Read the model definition and answer for the solid it produces. Units are mm, in the model's axes. Coordinates: 2 decimals unless noted, no trailing zeros. Order: outer loops, then holes, each group sorted by start corner. A loop starts at its lowest first (then second) coordinate and runs counter-clockwise, first axis right, second up. Notation, with made-up numbers: M 11,81.5 L 44,81.5 A22 cw 44,90.5 Z; hole C 51,-4.75 d9. An arc over 180 degrees is marked long. Use a Markdown table: item, result. Add a question column.
1) Find the intervals of material crossed by probe 1 along Y at (x, z) = (0, 22.75); probe 2 along X at (y, z) = (-40, 9.5); probe 3 along Y at (x, z) = (36.5, 10.25), in increasing order. Write a range as [from, to].
2) Find section B-B on x = -29.5. Write down the section's boundary in (y, z), plus the area to 3 significant figures.
3) Find section A-A on z = 3.75. Write down the section's boundary in (x, y), plus the area to 3 significant figures.
4) The mould has two halves that part along Y. Classify faces 1 (the face through (-43.3, 0.1, 14.8)), 2 (the face through (1.2, -20, 15)), 3 (the face through (-3, 0, 0)): released by +Y, released by -Y, zero draft, split by the parting line, or undercut.
5) Each of these flat-tipped pins is pushed along its axis until it touches: pin 1 Ø5 at (x, z) = (6.5, 17) entering from -Y; pin 2 Ø1 at (y, z) = (16.5, 24.5) entering from -X; pin 3 Ø12 at (y, z) = (10, 12.5) entering from +X. Where does it stop, or does it pass through?
from build123d import *

# Parameters (mm, degrees)
BOSS_EXTRUDE1_DEPTH = 30
SKETCH1_3_R         = 0.9
CUT_EXTRUDE1_DEPTH  = 30


with BuildPart() as part:
    # Sketch1 → Boss-Extrude1 (new body)
    with BuildSketch(Plane.XY):
        with BuildLine():
            Line((-1.2, -1.2), (-1.2, 0))
            Line((-1.2, 0), (-1.2, 1.2))
            Line((-1.2, 1.2), (-3.07408523, 1.2))
            ThreePointArc((-3.07408523, 1.2), (-3.3, 0), (-3.07408523, -1.2))
            Line((-3.07408523, -1.2), (-1.2, -1.2))
        make_face()
        with BuildLine():
            ThreePointArc((0, -1.2), (-0.848528137, -0.848528137), (-1.2, 0))
            Line((-1.2, 0), (-1.2, -1.2))
            Line((-1.2, -1.2), (0, -1.2))
        make_face()
        with BuildLine():
            ThreePointArc((0, 1.2), (-0.848528137, 0.848528137), (-1.2, 0))
            ThreePointArc((-1.2, 0), (-0.848528137, -0.848528137), (0, -1.2))
            ThreePointArc((0, -1.2), (0.848528137, -0.848528137), (1.2, 0))
            ThreePointArc((1.2, 0), (0.848528137, 0.848528137), (0, 1.2))
        make_face()
        with BuildLine():
            Line((-1.2, 1.2), (-1.2, 0))
            ThreePointArc((-1.2, 0), (-0.848528137, 0.848528137), (0, 1.2))
            Line((0, 1.2), (-1.2, 1.2))
        make_face()
        with BuildLine():
            Line((-3.07408523, 1.2), (-1.2, 1.2))
            Line((-1.2, 1.2), (-1.2, 3.07408523))
            ThreePointArc((-1.2, 3.07408523), (-2.333452378, 2.333452378), (-3.07408523, 1.2))
        make_face()
        with BuildLine():
            Line((-1.2, 3.07408523), (-1.2, 1.2))
            Line((-1.2, 1.2), (0, 1.2))
            Line((0, 1.2), (1.2, 1.2))
            Line((1.2, 1.2), (1.2, 3.07408523))
            ThreePointArc((1.2, 3.07408523), (0, 3.3), (-1.2, 3.07408523))
        make_face()
        with BuildLine():
            Line((0, -1.2), (-1.2, -1.2))
            Line((-1.2, -1.2), (-1.2, -3.07408523))
            ThreePointArc((-1.2, -3.07408523), (0, -3.3), (1.2, -3.07408523))
            Line((1.2, -3.07408523), (1.2, -1.2))
            Line((1.2, -1.2), (0, -1.2))
        make_face()
        with BuildLine():
            Line((-1.2, -3.07408523), (-1.2, -1.2))
            Line((-1.2, -1.2), (-3.07408523, -1.2))
            ThreePointArc((-3.07408523, -1.2), (-2.333452378, -2.333452378), (-1.2, -3.07408523))
        make_face()
        with BuildLine():
            ThreePointArc((1.2, 0), (0.848528137, -0.848528137), (0, -1.2))
            Line((0, -1.2), (1.2, -1.2))
            Line((1.2, -1.2), (1.2, 0))
        make_face()
        with BuildLine():
            Line((1.2, 1.2), (0, 1.2))
            ThreePointArc((0, 1.2), (0.848528137, 0.848528137), (1.2, 0))
            Line((1.2, 0), (1.2, 1.2))
        make_face()
        with BuildLine():
            Line((-1.2, 36.92591477), (-1.2, 3.07408523))
            ThreePointArc((-1.2, 3.07408523), (0, 3.3), (1.2, 3.07408523))
            Line((1.2, 3.07408523), (1.2, 36.92591477))
            ThreePointArc((1.2, 36.92591477), (0, 36.7), (-1.2, 36.92591477))
        make_face()
        with BuildLine():
            ThreePointArc((-3.07408523, -1.2), (-3.3, 0), (-3.07408523, 1.2))
            Line((-3.07408523, 1.2), (-36.92591477, 1.2))
            ThreePointArc((-36.92591477, 1.2), (-36.756970455, 0.610540229), (-36.7, 0))
            ThreePointArc((-36.7, 0), (-36.756970455, -0.610540229), (-36.92591477, -1.2))
            Line((-36.92591477, -1.2), (-3.07408523, -1.2))
        make_face()
        with BuildLine():
            ThreePointArc((1.2, -3.07408523), (0, -3.3), (-1.2, -3.07408523))
            Line((-1.2, -3.07408523), (-1.2, -36.92591477))
            ThreePointArc((-1.2, -36.92591477), (0, -36.7), (1.2, -36.92591477))
            Line((1.2, -36.92591477), (1.2, -3.07408523))
        make_face()
        with BuildLine():
            Line((1.2, 0), (1.2, -1.2))
            Line((1.2, -1.2), (3.07408523, -1.2))
            ThreePointArc((3.07408523, -1.2), (3.243029545, -0.610540229), (3.3, 0))
            ThreePointArc((3.3, 0), (3.243029545, 0.610540229), (3.07408523, 1.2))
            Line((3.07408523, 1.2), (1.2, 1.2))
            Line((1.2, 1.2), (1.2, 0))
        make_face()
        with BuildLine():
            Line((3.07408523, -1.2), (1.2, -1.2))
            Line((1.2, -1.2), (1.2, -3.07408523))
            ThreePointArc((1.2, -3.07408523), (2.333452378, -2.333452378), (3.07408523, -1.2))
        make_face()
        with BuildLine():
            Line((1.2, 3.07408523), (1.2, 1.2))
            Line((1.2, 1.2), (3.07408523, 1.2))
            ThreePointArc((3.07408523, 1.2), (2.333452378, 2.333452378), (1.2, 3.07408523))
        make_face()
        with BuildLine():
            ThreePointArc((3.3, 40), (-1.861451047, 42.724885319), (-1.2, 36.92591477))
            Line((-1.2, 36.92591477), (-1.2, 40))
            ThreePointArc((-1.2, 40), (0, 41.2), (1.2, 40))
            Line((1.2, 40), (1.2, 36.92591477))
            ThreePointArc((1.2, 36.92591477), (2.724885319, 38.138548953), (3.3, 40))
        make_face()
        with BuildLine():
            Line((-1.2, 40), (-1.2, 36.92591477))
            ThreePointArc((-1.2, 36.92591477), (0, 36.7), (1.2, 36.92591477))
            Line((1.2, 36.92591477), (1.2, 40))
            ThreePointArc((1.2, 40), (0, 41.2), (-1.2, 40))
        make_face()
        with BuildLine():
            ThreePointArc((-36.7, 0), (-36.756970455, 0.610540229), (-36.92591477, 1.2))
            Line((-36.92591477, 1.2), (-40, 1.2))
            ThreePointArc((-40, 1.2), (-41.2, 0), (-40, -1.2))
            Line((-40, -1.2), (-36.92591477, -1.2))
            ThreePointArc((-36.92591477, -1.2), (-36.756970455, -0.610540229), (-36.7, 0))
        make_face()
        with BuildLine():
            Line((-40, 1.2), (-36.92591477, 1.2))
            ThreePointArc((-36.92591477, 1.2), (-43.3, 0), (-36.92591477, -1.2))
            Line((-36.92591477, -1.2), (-40, -1.2))
            ThreePointArc((-40, -1.2), (-41.2, 0), (-40, 1.2))
        make_face()
        with BuildLine():
            ThreePointArc((1.2, -36.92591477), (0, -36.7), (-1.2, -36.92591477))
            Line((-1.2, -36.92591477), (-1.2, -40))
            ThreePointArc((-1.2, -40), (0, -41.2), (1.2, -40))
            Line((1.2, -40), (1.2, -36.92591477))
        make_face()
        with BuildLine():
            Line((-1.2, -40), (-1.2, -36.92591477))
            ThreePointArc((-1.2, -36.92591477), (-1.861451047, -42.724885319), (3.3, -40))
            ThreePointArc((3.3, -40), (2.724885319, -38.138548953), (1.2, -36.92591477))
            Line((1.2, -36.92591477), (1.2, -40))
            ThreePointArc((1.2, -40), (0, -41.2), (-1.2, -40))
        make_face()
        with BuildLine():
            ThreePointArc((3.3, 0), (3.243029545, -0.610540229), (3.07408523, -1.2))
            Line((3.07408523, -1.2), (36.92591477, -1.2))
            ThreePointArc((36.92591477, -1.2), (36.7, 0), (36.92591477, 1.2))
            Line((36.92591477, 1.2), (3.07408523, 1.2))
            ThreePointArc((3.07408523, 1.2), (3.243029545, 0.610540229), (3.3, 0))
        make_face()
        with BuildLine():
            ThreePointArc((36.92591477, 1.2), (36.7, 0), (36.92591477, -1.2))
            Line((36.92591477, -1.2), (40, -1.2))
            ThreePointArc((40, -1.2), (41.2, 0), (40, 1.2))
            Line((40, 1.2), (36.92591477, 1.2))
        make_face()
        with BuildLine():
            Line((40, -1.2), (36.92591477, -1.2))
            ThreePointArc((36.92591477, -1.2), (40.610540229, -3.243029545), (43.3, 0))
            ThreePointArc((43.3, 0), (40.610540229, 3.243029545), (36.92591477, 1.2))
            Line((36.92591477, 1.2), (40, 1.2))
            ThreePointArc((40, 1.2), (41.2, 0), (40, -1.2))
        make_face()
    extrude(amount=BOSS_EXTRUDE1_DEPTH)

    # Sketch1<3> → Cut-Extrude1 (cut)
    with BuildSketch(Plane.XY):
        Circle(SKETCH1_3_R)
        with Locations((0, 40)):
            Circle(SKETCH1_3_R)
        with Locations((40, 0)):
            Circle(SKETCH1_3_R)
        with Locations((0, -40)):
            Circle(SKETCH1_3_R)
        with Locations((-40, 0)):
            Circle(SKETCH1_3_R)
    extrude(amount=CUT_EXTRUDE1_DEPTH, mode=Mode.SUBTRACT)


solid = part.part
Check result:
| question | item | result |
|---|---|---|
| 1 | probe 1 | y = [-43.3, -40.9], [-39.1, -0.9], [0.9, 39.1], [40.9, 43.3] |
| 1 | probe 2 | x = [-3.3, -0.9], [0.9, 3.3] |
| 1 | probe 3 | y = [-1.2, 1.2] |
| 2 | outline | M -1.2,0 L 1.2,0 L 1.2,30 L -1.2,30 Z |
| 2 | area | 72.0 mm2 |
| 3 | outline | M -36.93,-1.2 L -3.07,-1.2 A3.3 ccw -1.2,-3.07 L -1.2,-36.93 A3.3 ccw long 1.2,-36.93 L 1.2,-3.07 A3.3 ccw 3.07,-1.2 L 36.93,-1.2 A3.3 ccw long 36.93,1.2 L 3.07,1.2 A3.3 ccw 1.2,3.07 L 1.2,36.93 A3.3 ccw long -1.2,36.93 L -1.2,3.07 A3.3 ccw -3.07,1.2 L -36.93,1.2 A3.3 ccw long Z; hole C -40,0 d1.8; hole C 0,-40 d1.8; hole C 0,0 d1.8; hole C 0,40 d1.8; hole C 40,0 d1.8 |
| 3 | area | 480 mm2 |
| 4 | face 1 | split by the parting line |
| 4 | face 2 | undercut |
| 4 | face 3 | zero draft |
| 5 | pin 1 | stops at y = -1.2 |
| 5 | pin 2 | stops at x = -1.2 |
| 5 | pin 3 | stops at x = 1.2 |
